Geometry: final body of the model. Coordinates: model frame, mm. Face numbers are marked on the shaded views. A direction names the side the tool comes from. Round coordinates to 2 decimals unless told otherwise and drop trailing zeros. Write each loop counter-clockwise with the first axis right and the second up, starting at its lowest first coordinate (ties: lowest second). Pieces come first, ordered by that corner, then holes. Notation, with made-up numbers: (-19, -34.75) -> (16, -34.75) arc R27 cw to (16, 1.25) -> close; hole circle Ø8 at (-7, -32). An arc over 180 degrees is marked (long way). Use one line per item in the form item = value. Start each with the question number.
1. Cut plane D-D, the plane z = -15.5. Return the cut outline in (x, y).
2. Cut plane A-A, the plane y = 9. Return the cut outline in (x, z), plus the area to 3 significant figures.
3. Pin query (flat end, axial travel): pin 1 Ø8 at (x, z) = (-4, -11) entering from +Y; pin 2 Ø1.8 at (x, y) = (0, 0) entering from +Z; pin 3 Ø12 at (x, y) = (-13.5, -13) entering from -Z. Return the tip coordinate at first contact, or that it passes through.
4. Cut plane C-C, the plane z = -9.25. Return the cut outline in (x, y), plus the area to 3 significant figures.
5. Cut plane B-B, the plane x = -3. Return the cut outline in (y, z).
6. Line query: L1, parallel to X at y = 0, z = -4.25; L2, parallel to Y at x = 0, z = -7. Output: solid intervals per line, ascending.
7. Reachability of the marked faces 1 and 2 from +Z, -Z, +X, -X, +Y, -Y: full face, straight path, thin tool, end or side. Return the list, or none.
```python
from build123d import *

# Parameters (mm, degrees)
F0_W     = 35
F0_H     = 35
F1_DEPTH = 6
F4_D     = 3
F4_DEPTH = 10
F4_TIP   = 0.9012909285


with BuildPart() as f1:
    # F0 (on Top) → F1 (new body)
    with BuildSketch(Plane.XY):
        Rectangle(F0_W, F0_H)
    extrude(amount=-F1_DEPTH)

    # F2 (on Front) → F3 (revolve)
    with BuildSketch(Plane.XZ):
        with BuildLine():
            Line((0, -6), (0, -21))
            ThreePointArc((0, -21), (10.6066017178, -16.6066017178), (15, -6))
            Line((15, -6), (0, -6))
        make_face()
    revolve(axis=Axis((0, 0, -13.5), (0, 0, -1)))

    # F4
    with Locations(Plane.XY):
        with Locations((0, 0)):
            Hole(F4_D / 2, depth=F4_DEPTH)
            with Locations((0, 0, -(F4_DEPTH + F4_TIP / 2))):  # 118° drill point
                Cone(0, F4_D / 2, F4_TIP, mode=Mode.SUBTRACT)


solid = f1.part
```
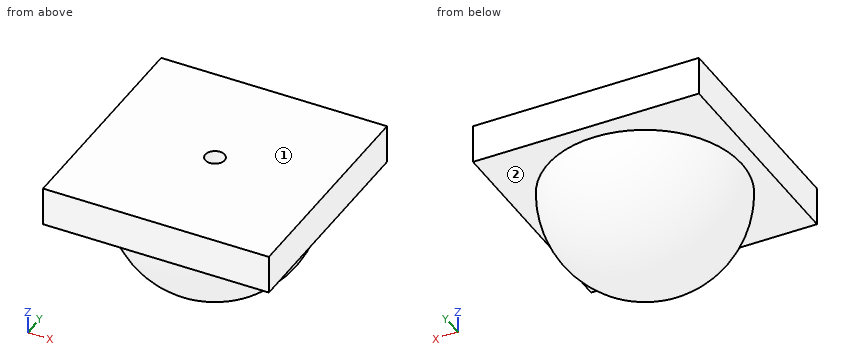
Outcome:
q1.outline = circle Ø23.22 at (0, 0)
q2.outline = (-17.5, -6) -> (-12, -6) arc R12 ccw to (12, -6) -> (17.5, -6) -> (17.5, 0) -> (-17.5, 0) -> close
q2.area = 436 mm^2
q3.pin_1 = 14.81
q3.pin_2 = -10.36
q3.pin_3 = -13.92
q4.outline = circle Ø29.29 at (0, 0); hole circle Ø3 at (0, 0)
q4.area = 667 mm^2
q5.outline = (-17.5, -6) -> (-14.7, -6) arc R14.7 ccw to (14.7, -6) -> (17.5, -6) -> (17.5, 0) -> (-17.5, 0) -> close
q6.L1 = -17.5 to -1.5, 1.5 to 17.5
q6.L2 = -14.97 to -1.5, 1.5 to 14.97
q7.face_1 = +Z, +X, -X, +Y, -Y
q7.face_2 = -Z
